CAD build for the part. Positions are in the model's coordinates, mm. Face numbers are marked on the shaded views. A direction names the side the tool comes from. Round coordinates to 2 decimals unless told otherwise and drop trailing zeros. Loops run counter-clockwise (first coordinate to the right, second up) from the corner with the lowest first, then second, coordinate; pieces in that order, holes last.
```python
from build123d import *

# Parameters (mm, degrees)
SKETCH1_W                = 19.9
SKETCH1_H                = 8.6
SKETCH1_R                = 1.2
BOSS_EXTRUDE1_DEPTH      = 0.79375
CONVERT_SOLID2_START     = -0.79375
CONVERT_SOLID2_OUTLINE_W = 19.9
CONVERT_SOLID2_OUTLINE_H = 8.6
CONVERT_SOLID2_OUTLINE_R = 1.2
CONVERT_SOLID2_DEPTH     = 0.79375
EDGE_FLANGE1_DEPTH       = 19.9
EDGE_FLANGE2_DEPTH       = 19.9
EDGE_FLANGE2_START       = 1.5875
EDGE_FLANGE2_PROFILE_W   = 19.9
EDGE_FLANGE2_PROFILE_H   = 8.6
EDGE_FLANGE2_PROFILE_R   = 1.2
EDGE_FLANGE2_FLAT_DEPTH  = 1.5875


# Read off the part's stored shape, not the designer's step: Convert-Solid2
# Sheet-metal steps are written as plain solids
with BuildPart() as part:
    # Sketch1 → Boss-Extrude1 (new body)
    with BuildSketch(Plane.XY):
        with Locations((0, -1.76)):
            Rectangle(SKETCH1_W, SKETCH1_H)
        with Locations((-4.75, 0)):
            Circle(SKETCH1_R, mode=Mode.SUBTRACT)
        with Locations((4.75, 0)):
            Circle(SKETCH1_R, mode=Mode.SUBTRACT)
    extrude(amount=BOSS_EXTRUDE1_DEPTH)

    # Convert-Solid2 outline → Convert-Solid2 (add)
    with BuildSketch(Plane.XY.offset(CONVERT_SOLID2_START)):
        with Locations((0, -1.76)):
            Rectangle(CONVERT_SOLID2_OUTLINE_W, CONVERT_SOLID2_OUTLINE_H)
        with Locations((-4.75, 0)):
            Circle(CONVERT_SOLID2_OUTLINE_R, mode=Mode.SUBTRACT)
        with Locations((4.75, 0)):
            Circle(CONVERT_SOLID2_OUTLINE_R, mode=Mode.SUBTRACT)
    extrude(amount=CONVERT_SOLID2_DEPTH)

    # Edge-Flange1 section (across the edge) → Edge-Flange1 (add)
    with BuildSketch(Plane(origin=(9.95, -7.33, -0.79375), x_dir=(0, 1, 0), z_dir=(-1, 0, 0))):
        with BuildLine():
            Line((-1.5875, 1.27), (-1.5875, 10))
            Line((-1.5875, 10), (0, 10))
            Line((0, 10), (0, 1.27))
            ThreePointArc((0, 1.27), (0.371974388, 0.371974388), (1.27, 0))
            Line((1.27, 0), (1.27, -1.5875))
            ThreePointArc((1.27, -1.5875), (-0.750557627, -0.750557627), (-1.5875, 1.27))
        make_face()
    extrude(amount=EDGE_FLANGE1_DEPTH)

    # Edge-Flange2 bend section (across the edge) → Edge-Flange2 (add)
    with BuildSketch(Plane(origin=(9.95, -7.33, -11.79375), x_dir=(0, 0, 1), z_dir=(-1, 0, 0))):
        with BuildLine():
            Line((-1.5875, 1), (0, 1))
            ThreePointArc((0, 1), (0.292893219, 0.292893219), (1, 0))
            Line((1, 0), (1, -1.5875))
            ThreePointArc((1, -1.5875), (-0.829638796, -0.829638796), (-1.5875, 1))
        make_face()
    extrude(amount=EDGE_FLANGE2_DEPTH)

    # Edge-Flange2 profile (on flange) → Edge-Flange2 flat (add)
    with BuildSketch(Plane(origin=(0, -7.33, -11.79375), x_dir=(-1, 0, 0), z_dir=(0, 0, -1)).offset(EDGE_FLANGE2_START)):
        with Locations((0, 5.3)):
            Rectangle(EDGE_FLANGE2_PROFILE_W, EDGE_FLANGE2_PROFILE_H)
        with Locations((-4.75, 7.06)):
            Circle(EDGE_FLANGE2_PROFILE_R, mode=Mode.SUBTRACT)
        with Locations((4.75, 7.06)):
            Circle(EDGE_FLANGE2_PROFILE_R, mode=Mode.SUBTRACT)
    extrude(amount=-EDGE_FLANGE2_FLAT_DEPTH)


solid = part.part
```
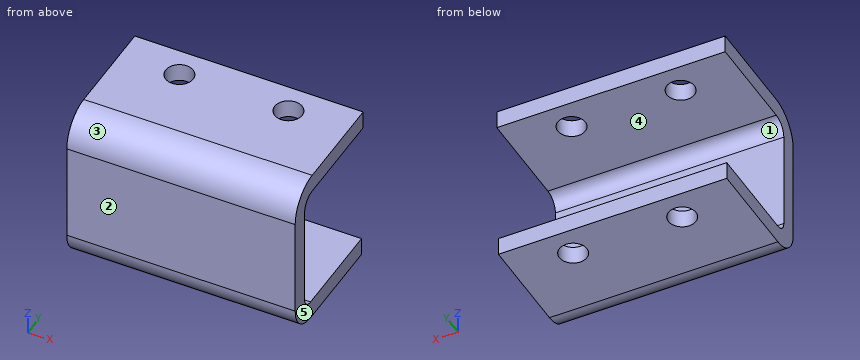
Item 1: Cut at C-C, the plane y = -0.27. Give the cut face in (x, z), plus the area to 3 significant figures.
Answers follow:
outline: (-9.95, -13.38) - (-5.95, -13.38) - (-5.95, -11.79) - (-9.95, -11.79) - close; (-9.95, -0.79) - (-5.92, -0.79) - (-5.92, 0.79) - (-9.95, 0.79) - close; (-3.58, -0.79) - (3.58, -0.79) - (3.58, 0.79) - (-3.58, 0.79) - close; (-3.55, -13.38) - (3.55, -13.38) - (3.55, -11.79) - (-3.55, -11.79) - close; (5.92, -0.79) - (9.95, -0.79) - (9.95, 0.79) - (5.92, 0.79) - close; (5.95, -13.38) - (9.95, -13.38) - (9.95, -11.79) - (5.95, -11.79) - close
area: 48.1 mm2
Item 2: Two-plate mould, pull along Z, no slides. Class the marked faces 1, 2 and 3: released by +Z, released by -Z, zero draft, split by the parting line, or undercut.
Answers follow:
face 1: undercut
face 2: zero draft
face 3: released by +Z
Item 3: Cut at A-A, the plane y = -3.5. Give the cut face in (x, z), plus the area to 3 significant figures.
Answers follow:
outline: (-9.95, -13.38) - (9.95, -13.38) - (9.95, -11.79) - (-9.95, -11.79) - close; (-9.95, -0.79) - (9.95, -0.79) - (9.95, 0.79) - (-9.95, 0.79) - close
area: 63.2 mm2
Item 4: Probe line 1 (Z direction, x = -5.75, y = -3.25); line 2 (Y direction, x = -8, z = -2.75); line 3 (Y direction, x = -4.75, z = -12.2). List the from-to ranges inside material, lowest first.
Answers follow:
line 1: z = -13.38 to -11.79, -0.79 to 0.79
line 2: y = -8.92 to -7.33
line 3: y = -8.5 to -1.47, 0.93 to 2.27
Item 5: Flat gauge pin, fed straight in: P1, Ø7, axis at x = 3, z = -8.5, coming from the +Y side. Where does the tip first touch, or does it go through?
Answers follow:
P1: stops at y = 2.27
Item 6: Cut at B-B, the plane x = 4.75. Give the cut face in (y, z) (1 decimal).
Answers follow:
outline: (-8.9, -10.8) arc R2.6 ccw to (-6.3, -13.4) - (-1.5, -13.4) - (-1.5, -11.8) - (-6.3, -11.8) arc R1 cw to (-7.3, -10.8) - (-7.3, -2.1) arc R1.3 cw to (-6.1, -0.8) - (-1.2, -0.8) - (-1.2, 0.8) - (-6.1, 0.8) arc R2.9 ccw to (-8.9, -2.1) - close; (0.9, -13.4) - (2.3, -13.4) - (2.3, -11.8) - (0.9, -11.8) - close; (1.2, -0.8) - (2.5, -0.8) - (2.5, 0.8) - (1.2, 0.8) - close
Item 7: 3-axis set-ups, long thin cutter, end or side, ignore diameter. For the marked faces 4 and 5: which of +Z, -Z, +X, -X, +Y, -Y reach the whole face in a straight line?
Answers follow:
face 4: +X, -X, +Y
face 5: +Z, -Z, +X, +Y, -Y
Item 8: Cut at D-D, the plane x = 2.5. Give the cut face in (y, z) (1 decimal), plus the area to 3 significant figures.
Answers follow:
outline: (-8.9, -10.8) arc R2.6 ccw to (-6.3, -13.4) - (2.3, -13.4) - (2.3, -11.8) - (-6.3, -11.8) arc R1 cw to (-7.3, -10.8) - (-7.3, -2.1) arc R1.3 cw to (-6.1, -0.8) - (2.5, -0.8) - (2.5, 0.8) - (-6.1, 0.8) arc R2.9 ccw to (-8.9, -2.1) - close
area: 50.8 mm2
